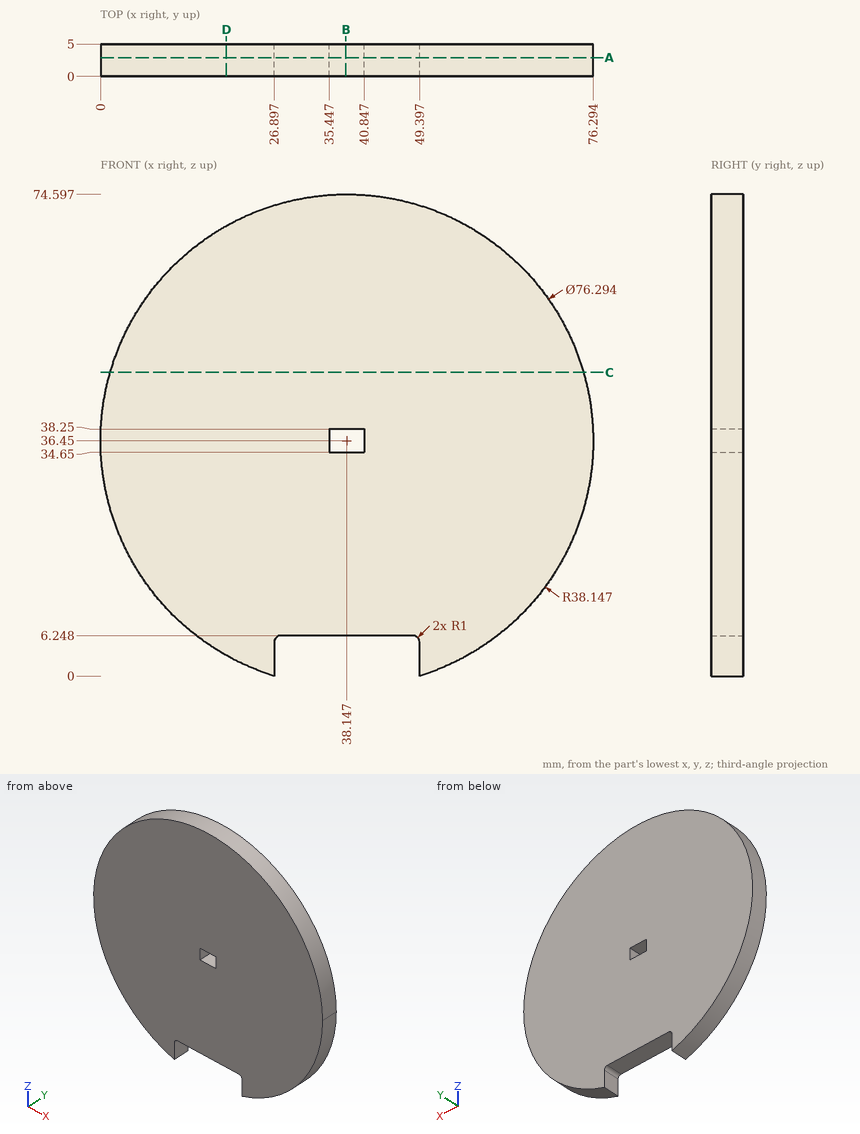
Check sheet for the drawn part. Datum: minimum x, y, z corner. Units: mm. Round coordinates to 2 decimals unless told otherwise and drop trailing zeros. Loops run counter-clockwise (first coordinate to the right, second up) from the corner with the lowest first, then second, coordinate; pieces in that order, holes last. Notation, with made-up numbers: (68, -0.5) -> (121, -0.5) arc R15 ccw to (121, 17.5) -> close; hole circle Ø1 at (69, -10.75). An arc over 180 degrees is marked (long way). Put each result on its own line as item: value. Start each with the question number.
1. Section check B-B (x = 38). Enter the section's corners in (y, z).
2. Scan lines: probe 1 along Z at (x, y) = (36, 1.6); probe 2 along X at (y, z) = (2.65, 67.5) (1 decimal); probe 3 along X at (y, z) = (1.65, 5) (1 decimal). Record each from-to range of solid material in increasing order.
3. Section check D-D (x = 19.5). Enter the section's corners in (y, z).
4. Section check A-A (y = 2.9). Enter the section's corners in (x, z), plus the area to 3 significant figures.
5. Gauge pin test, flat ends, axial feed: pin 1 (1.8 mm diameter, centred on y = 3, z = 36.5, fed in from -X); pin 2 (1 mm diameter, centred on x = 16.5, y = 3, fed in from -Z); pin 3 (3 mm diameter, centred on x = 36.5, y = 1, fed in from -Z). Record the tip position at first contact, or that the pin passes through.
6. Section check C-C (z = 47). Enter the section's corners in (x, y).
Findings:
1. outline: (0, 6.25) -> (5, 6.25) -> (5, 34.65) -> (0, 34.65) -> close; (0, 38.25) -> (5, 38.25) -> (5, 74.6) -> (0, 74.6) -> close
2. probe 1: z = 6.25 to 34.65, 38.25 to 74.54
2. probe 2: x = 16 to 60.3
2. probe 3: x = 16.6 to 26.9, 49.4 to 59.7
3. outline: (0, 3.17) -> (5, 3.17) -> (5, 69.73) -> (0, 69.73) -> close
4. outline: (26.9, 0) -> (26.9, 5.25) arc R1 cw to (27.9, 6.25) -> (48.4, 6.25) arc R1 cw to (49.4, 5.25) -> (49.4, 0) arc R38.15 ccw (long way) to start; hole (35.45, 34.65) -> (40.85, 34.65) -> (40.85, 38.25) -> (35.45, 38.25) -> close
4. area: 4,390 mm^2
5. pin 1: stops at x = 0
5. pin 2: stops at z = 4.7
5. pin 3: stops at z = 6.25
6. outline: (1.49, 0) -> (74.81, 0) -> (74.81, 5) -> (1.49, 5) -> close
